from build123d import *

# Parameters (mm, degrees)
F0_R     = 15
F1_DEPTH = 4
F2_T     = -1
F3_R     = 7
F4_DEPTH = 1.1


with BuildPart() as f1:
    # F0 (on Top) → F1 (new body)
    with BuildSketch(Plane.XY):
        Circle(F0_R)
    extrude(amount=F1_DEPTH)

    # F2
    f2_openings = [f1.faces().sort_by_distance(p)[0] for p in [
        (0, 0, 4),
    ]]
    offset(amount=F2_T, openings=f2_openings)

    # F3 (on Top) → F4 (cut)
    with BuildSketch(Plane.XY):
        Circle(F3_R)
    extrude(amount=F4_DEPTH, mode=Mode.SUBTRACT)


solid = f1.part
Could you check a few things on this model? Use its own coordinates, in mm. A direction names the side the tool comes from. Coordinates: 2 decimals unless noted, no trailing zeros. Loops run counter-clockwise (first coordinate to the right, second up) from the corner with the lowest first, then second, coordinate; pieces in that order, holes last.
1. Imagine slicing it at C-C (z = 0.5). Please give me the cut outline in (x, y), and give its area (3 significant figures).
2. For faces 1 (the face through (-6.4, 3.3, 1)), 2 (the face through (6.466, -2.681, 0.493)), which set-ups out of +Z, -Z, +X, -X, +Y, -Y let a thin tool reach every point of the face, with its end or its side?
3. Imagine slicing it at D-D (x = -12). Please give me the cut outline in (y, z), and give its area (3 significant figures).
4. Imagine slicing it at A-A (y = 0). Please give me the cut outline in (x, z).
5. For P1, Ø5, axis at x = 0, y = -5.5, coming from the +Z side; P2, Ø1, axis at x = 7, z = 1, coming from the -Y side, each with a flat end and sliding along its axis, tell me the tip position at first contact or that it passes through.
6. I need wall thicknesses on L1, parallel to Y at x = 0, z = 0.8; L2, parallel to Y at x = 0, z = 2.1. Which ranges of each line are inside material? Lowest first, please.
Computed values:
1. outline: circle Ø30 at (0, 0); hole circle Ø14 at (0, 0)
1. area: 553 mm2
2. face 1: +Z
2. face 2: +Z, -Z
3. outline: (-9, 0) - (9, 0) - (9, 4) - (7.21, 4) - (7.21, 1) - (-7.21, 1) - (-7.21, 4) - (-9, 4) - close
3. area: 28.7 mm2
4. outline: (-15, 0) - (-7, 0) - (-7, 1) - (-14, 1) - (-14, 4) - (-15, 4) - close; (7, 0) - (15, 0) - (15, 4) - (14, 4) - (14, 1) - (7, 1) - close
5. P1: stops at z = 1
5. P2: stops at y = -13.52
6. L1: y = -15 to -7, 7 to 15
6. L2: y = -15 to -14, 14 to 15
